Model file for the job. Use its own axes, mm. Round coordinates to 2 decimals unless told otherwise and drop trailing zeros. Order: outer loops, then holes, each group sorted by start corner. A loop starts at its lowest first (then second) coordinate and runs counter-clockwise, first axis right, second up. Notation, with made-up numbers: (56.5, -9) - (94.5, -9) arc R35 ccw to (94.5, 30) - close; hole circle Ø7 at (-5, 5.5). An arc over 180 degrees is marked (long way). Write item = value, one per line. Start each with the question number.
Autodesk Inventor part; units mm, degrees
ref_plane "YZ Plane" through (0, 0, 0) normal (1, 0, 0) x (0, 1, 0)
ref_plane "XZ Plane" through (0, 0, 0) normal (0, 1, 0) x (-1, 0, 0)
ref_plane "XY Plane" through (0, 0, 0) normal (0, 0, 1) x (1, 0, 0)
sketch "草圖1" plane through (0, 0, 0) normal (0, 1, 0) x (-1, 0, 0)
  line L0 (140, 0) -> (0, 0)
  line L1 (0, 0) -> (0, -290)
  line L2 (0, -290) -> (140, -290)
  line L3 (140, -290) -> (140, 0)
  line L4 (0, 0) -> (8, 0)
  line L5 (8, 0) -> (8, -40)
  line L6 (8, -40) -> (0, -40)
  line L7 (0, -40) -> (0, 0)
  line L8 (140, 0) -> (132, 0)
  line L9 (132, 0) -> (132, -40)
  line L10 (132, -40) -> (140, -40)
  line L11 (140, -40) -> (140, 0)
  line L12 (140, -290) -> (132, -290)
  line L13 (132, -290) -> (132, -250)
  line L14 (132, -250) -> (140, -250)
  line L15 (140, -250) -> (140, -290)
  line L16 (0, -290) -> (8, -290)
  line L17 (8, -290) -> (8, -250)
  line L18 (8, -250) -> (0, -250)
  line L19 (0, -250) -> (0, -290)
  line L20 (140, -131.5) -> (88, -131.5)
  line L21 (88, -131.5) -> (88, -158.5)
  line L22 (88, -158.5) -> (140, -158.5)
  line L23 (140, -158.5) -> (140, -131.5)
  line L24 (52, -131.5) -> (0, -131.5)
  line L25 (0, -131.5) -> (0, -158.5)
  line L26 (0, -158.5) -> (52, -158.5)
  line L27 (52, -158.5) -> (52, -131.5)
  point P0 (140, -145)
  point P1 (0, -145)
  point P2 (0, -40)
  point P3 (0, -131.5)
  point P4 (0, -158.5)
  point P5 (0, -250)
  point P6 (132, -290)
  dimension "d0" = 140
  dimension "d1" = 290
  dimension "d2" = 8
  dimension "d3" = 40
  dimension "d4" = 52
  dimension "d5" = 27
extrude "擠出1" add sketch "草圖1" along normal blind 10 contours L9 L10 L3 L20 L21 L22 L14 L13 L2 L17 L18 L1 L26 L27 L24 L6 L5 L0
properties part number "plate"
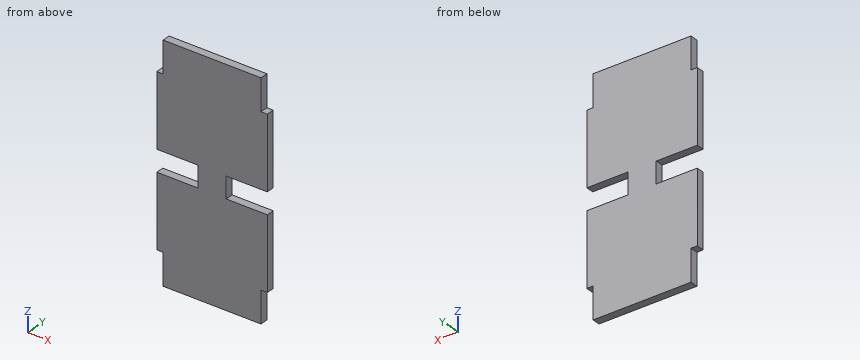
Item 1: Saw through at C-C, the plane z = -33. Give the cut face in (x, y), then the cut area to 3 significant figures.
Item 2: Saw through at A-A, the plane x = -16. Give the cut face in (y, z), then the cut area to 3 significant figures.
Item 3: Saw through at B-B, the plane y = 2.75. Give the cut face in (x, z), then the cut area to 3 significant figures.
Item 4: Probe L1, parallel to Z at x = -11.5, y = 9.5; L2, parallel to X at y = 3, z = -143.5; L3, parallel to X at y = 8, z = -35. List the from-to ranges inside material, lowest first.
Item 5: Drop flat-ended pins along their axis: pin 1 (5 mm diameter, centred on y = 3, z = -269.5, fed in from -X); pin 2 (3 mm diameter, centred on y = 3, z = -274, fed in from +X); pin 3 (4 mm diameter, centred on x = -135, y = 2.5, fed in from +Z). Give the stop position or say it passes through.
Item 6: Saw through at D-D, the plane z = -142. Give the cut face in (x, y).
Check sheet entries:
q1.outline = (-132, 0) - (-8, 0) - (-8, 10) - (-132, 10) - close
q1.area = 1,240 mm2
q2.outline = (0, -290) - (10, -290) - (10, -158.5) - (0, -158.5) - close; (0, -131.5) - (10, -131.5) - (10, 0) - (0, 0) - close
q2.area = 2,630 mm2
q3.outline = (-140, -250) - (-132, -250) - (-132, -290) - (-8, -290) - (-8, -250) - (0, -250) - (0, -158.5) - (-52, -158.5) - (-52, -131.5) - (0, -131.5) - (0, -40) - (-8, -40) - (-8, 0) - (-132, 0) - (-132, -40) - (-140, -40) - (-140, -131.5) - (-88, -131.5) - (-88, -158.5) - (-140, -158.5) - close
q3.area = 36,500 mm2
q4.L1 = -290 to -158.5, -131.5 to 0
q4.L2 = -88 to -52
q4.L3 = -132 to -8
q5.pin_1 = -132
q5.pin_2 = -8
q5.pin_3 = -40
q6.outline = (-88, 0) - (-52, 0) - (-52, 10) - (-88, 10) - close
